from build123d import *

# Parameters (mm, degrees)
IZIM2_R                              = 8
IZIM2_R_2                            = 11
Y_KSEKLIK_EKSTR_ZYON1_DEPTH          = 24
M4_HELISARMAL_I_IN_Z_VANA_MATKAB_1_D = 4.2


with BuildPart() as part:
    # Çizim2 → Yükseklik-Ekstrüzyon1 (new body)
    with BuildSketch(Plane.XY):
        with BuildLine():
            Line((-52.954462088, 36.177194256), (69.725029836, 36.177194256))
            ThreePointArc((69.725029836, 36.177194256), (74.055156855, 33.677194256), (74.055156855, 28.677194256))
            Line((74.055156855, 28.677194256), (12.715410893, -77.566362274))
            ThreePointArc((12.715410893, -77.566362274), (8.385283874, -80.066362274), (4.055156855, -77.566362274))
            Line((4.055156855, -77.566362274), (-57.284589107, 28.677194256))
            ThreePointArc((-57.284589107, 28.677194256), (-57.284589107, 33.677194256), (-52.954462088, 36.177194256))
        make_face()
        with Locations((57.600674183, 24.177194256)):
            Circle(IZIM2_R, mode=Mode.SUBTRACT)
        with Locations((8.385283874, -61.066362274)):
            Circle(IZIM2_R, mode=Mode.SUBTRACT)
        with Locations((-40.830106435, 24.177194256)):
            Circle(IZIM2_R, mode=Mode.SUBTRACT)
        with Locations((8.385283874, -4.237324587)):
            Circle(IZIM2_R_2, mode=Mode.SUBTRACT)
    extrude(amount=Y_KSEKLIK_EKSTR_ZYON1_DEPTH)

    # M4 Helisarmal için Zıvana matkabı1 (through all)
    with Locations(Plane(origin=(-16.222411281, 9.969934834, 24), x_dir=(1, 0, 0), z_dir=(0, 0, 1))):
        with Locations((0, 0), (49.215390309, 0), (24.607695155, -42.621778265)):
            Hole(M4_HELISARMAL_I_IN_Z_VANA_MATKAB_1_D / 2)


solid = part.part
Input: part model. Units: mm. Frame: model coordinates. Round coordinates to 2 decimals unless told otherwise and drop trailing zeros. Order: outer loops, then holes, each group sorted by start corner. A loop starts at its lowest first (then second) coordinate and runs counter-clockwise, first axis right, second up. Notation, with made-up numbers: (16, -20.5) - (40, -20.5) arc R24 cw to (40, 16.5) - close; hole circle Ø6 at (-15.5, 59). An arc over 180 degrees is marked (long way). Use a Markdown table: item, result.
1. First-contact query: pin 1 (2 mm diameter, centred on y = -43, z = 20.5, fed in from -X); pin 2 (12 mm diameter, centred on y = -4.5, z = 8.5, fed in from -X); pin 3 (5 mm diameter, centred on y = 6.5, z = 11.5, fed in from +X). Flat tips, straight axial feed; report the tip coordinate or a pass-through.
Evaluation:
| item | result |
|---|---|
| pin 1 | x = -16.48 |
| pin 2 | x = -41.59 |
| pin 3 | x = 62.69 |
2. Mould query, pull axis X, two halves, no side actions, for faces 1 (the face through (43.815, -23.701, 11.832)), 2 (the face through (8.84, -34.7, 11.83)), 3 (the face through (-57.321, 33.613, 11.832)), 4 (the face through (8, 36.177, 12)). Classes: +X half, -X half, draft (parallel to the pull), parting line (faces both ways), or undercut.
Evaluation:
| item | result |
|---|---|
| face 1 | +X half |
| face 2 | undercut |
| face 3 | -X half |
| face 4 | draft |
3. Section B-B on z = 12.5. Return the cut outline in (x, y), then the cut area to 3 significant figures.
Evaluation:
| item | result |
|---|---|
| outline | (-57.28, 28.68) - (4.06, -77.57) arc R5 ccw to (12.72, -77.57) - (74.06, 28.68) arc R5 ccw to (69.73, 36.18) - (-52.95, 36.18) arc R5 ccw to start; hole circle Ø16 at (-40.83, 24.18); hole circle Ø4.2 at (-16.22, 9.97); hole circle Ø22 at (8.39, -4.24); hole circle Ø16 at (8.39, -61.07); hole circle Ø4.2 at (8.39, -32.65); hole circle Ø4.2 at (32.99, 9.97); hole circle Ø16 at (57.6, 24.18) |
| area | 7,410 mm^2 |
4. Section A-A on x = -41.5. Return the cut outline in (y, z).
Evaluation:
| item | result |
|---|---|
| outline | (1.34, 0) - (16.21, 0) - (16.21, 24) - (1.34, 24) - close; (32.15, 0) - (36.18, 0) - (36.18, 24) - (32.15, 24) - close |
5. Section C-C on y = -55.5. Return the cut outline in (x, z), then the cut area to 3 significant figures.
Evaluation:
| item | result |
|---|---|
| outline | (-8.68, 0) - (2.64, 0) - (2.64, 24) - (-8.68, 24) - close; (14.13, 0) - (25.46, 0) - (25.46, 24) - (14.13, 24) - close |
| area | 544 mm^2 |
6. Material intervals for probe 1 along X at (y, z) = (23, 7.5); probe 2 along Y at (x, z) = (2.5, 7.75); probe 3 along Y at (x, z) = (12, 2.75), sorted ascending.
Evaluation:
| item | result |
|---|---|
| probe 1 | -54.01 to -48.74, -32.92 to 49.69, 65.51 to 70.78 |
| probe 2 | -74.87 to -66.49, -55.65 to -13.53, 5.06 to 36.18 |
| probe 3 | -78.52 to -68.2, -53.93 to -14.63, 6.15 to 36.18 |
7. Section D-D on x = 8.5. Return the cut outline in (y, z).
Evaluation:
| item | result |
|---|---|
| outline | (-80.07, 0) - (-69.07, 0) - (-69.07, 24) - (-80.07, 24) - close; (-53.07, 0) - (-34.75, 0) - (-34.75, 24) - (-53.07, 24) - close; (-30.55, 0) - (-15.24, 0) - (-15.24, 24) - (-30.55, 24) - close; (6.76, 0) - (36.18, 0) - (36.18, 24) - (6.76, 24) - close |
